from build123d import *

# Parameters (mm, degrees)
SKETCH3_R          = 1.75
CUT_EXTRUDE1_DEPTH = 10
SKETCH5_W          = 10
SKETCH5_H          = 10
CUT_EXTRUDE3_DEPTH = 50
CHAMFER1_START     = -23
CHAMFER1_2_DEPTH   = 2


with BuildPart() as part:
    # Sketch2 → Revolve1 (revolve)
    with BuildSketch(Plane.XY, mode=Mode.PRIVATE) as revolve1_sk:
        Polygon((25.1, 13), (27.1, 13), (27.1, -24), (37.1, -24), (37.1, -27), (24.1, -27), (24.1, -13), (25.1, -13), align=None)
    revolve(revolve1_sk.sketch.rotate(Axis((0, 0, 0), (0, -1, 0)), 90), axis=Axis((0, 0, 0), (0, -1, 0)))

    # Sketch3 → Cut-Extrude1 (cut)
    with BuildSketch(Plane(origin=(0, -24, 0), x_dir=(1, 0, 0), z_dir=(0, 1, 0))):
        with Locations(Location((-23.228457762, 23.228457762, 0), (0, 0, 270))):
            Circle(SKETCH3_R)
        with Locations(Location((23.228457762, 23.228457762, 0), (0, 0, 270))):
            Circle(SKETCH3_R)
        with Locations(Location((23.228457762, -23.228457762, 0), (0, 0, 270))):
            Circle(SKETCH3_R)
        with Locations(Location((-23.228457762, -23.228457762, 0), (0, 0, 270))):
            Circle(SKETCH3_R)
    extrude(amount=-CUT_EXTRUDE1_DEPTH, mode=Mode.SUBTRACT)

    # Sketch5 → Cut-Extrude3 (cut)
    with BuildSketch(Plane.XY):
        with Locations((0, -18)):
            Rectangle(SKETCH5_W, SKETCH5_H)
    extrude(amount=-CUT_EXTRUDE3_DEPTH, mode=Mode.SUBTRACT)

    # Chamfer1: read off the stored shape, not the designer's step
    # Chamfer1 outline → Chamfer1 (revolve)
    with BuildSketch(Plane.XY):
        Polygon((29.1, -24), (27.1, -22), (27.1, -24), align=None)
    revolve(axis=Axis((0, 0, 0), (0, 1, 0)))

    # Chamfer1 2 outline → Chamfer1 2 (cut)
    with BuildSketch(Plane(origin=(0, 0, 0), x_dir=(1, 0, 0), z_dir=(0, 1, 0)).offset(CHAMFER1_START)):
        with BuildLine():
            ThreePointArc((5, 27.651582233), (0, 28.1), (-5, 27.651582233))
            Line((-5, 27.651582233), (-5, 23.575623003))
            ThreePointArc((-5, 23.575623003), (0, 24.1), (5, 23.575623003))
            Line((5, 23.575623003), (5, 27.651582233))
        make_face()
    extrude(amount=CHAMFER1_2_DEPTH, mode=Mode.SUBTRACT)


solid = part.part
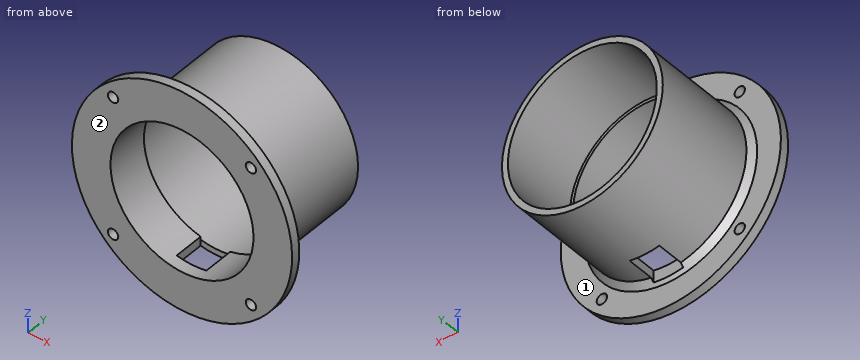
Design review of the part built by this model. Coordinates are the model's own, in mm. Face numbers are marked on the shaded views. A direction names the side the tool comes from. Coordinates: 2 decimals unless noted, no trailing zeros. Write each loop counter-clockwise with the first axis right and the second up, starting at its lowest first coordinate (ties: lowest second). Pieces come first, ordered by that corner, then holes. Notation, with made-up numbers: (83, -1.5) - (116, -1.5) arc R3 cw to (116, 2.5) - close; hole circle Ø2 at (-11, -21.5). An arc over 180 degrees is marked (long way). Use one line per item in the form item = value.
Q1. Consider section C-C (y = 1.5). Write out the cut boundary in (x, z).
Taken from the geometry:
outline = circle Ø54.2 at (0, 0); hole circle Ø50.2 at (0, 0)
Q2. Machinability: for the marked faces 1 and 2, which of the approach directions +Z, -Z, +X, -X, +Y, -Y give a long, thin tool a straight path to every point of the face, cutting with its end or side? Answer none if there is none.
Taken from the geometry:
face_1 = +Y
face_2 = +Z, -Z, +X, -X, -Y
Q3. Consider section B-B (x = 0). Write out the cut boundary in (y, z).
Taken from the geometry:
outline = (-27, -37.1) - (-24, -37.1) - (-24, -29.1) - (-23, -28.1) - (-23, -24.1) - (-27, -24.1) - close; (-27, 24.1) - (-13, 24.1) - (-13, 25.1) - (13, 25.1) - (13, 27.1) - (-22, 27.1) - (-24, 29.1) - (-24, 37.1) - (-27, 37.1) - close; (-13, -27.1) - (13, -27.1) - (13, -25.1) - (-13, -25.1) - close
Q4. Consider section A-A (z = 0). Write out the cut boundary in (x, y), plus the area to 3 significant figures.
Taken from the geometry:
outline = (-37.1, -27) - (-24.1, -27) - (-24.1, -13) - (-25.1, -13) - (-25.1, 13) - (-27.1, 13) - (-27.1, -22) - (-29.1, -24) - (-37.1, -24) - close; (24.1, -27) - (37.1, -27) - (37.1, -24) - (29.1, -24) - (27.1, -22) - (27.1, 13) - (25.1, 13) - (25.1, -13) - (24.1, -13) - close
area = 252 mm^2
Q5. For probe 1 along Z at (x, y) = (-0.5, -0.5); probe 2 along Y at (x, z) = (25, -23); probe 3 along X at (y, z) = (-20, -12.5), list the stretches that pass through material, from the lowest coordinate up.
Taken from the geometry:
probe_1 = -27.1 to -25.1, 25.1 to 27.1
probe_2 = -27 to -24
probe_3 = -24.04 to -20.6, 20.6 to 24.04
Q6. Insertion check: pin 1 Ø1.5 at (x, y) = (22.5, -4) entering from -Z; pin 2 Ø3 at (x, y) = (-19.5, -19) entering from +Z; pin 3 Ø4 at (x, z) = (-23.23, -23.23) entering from +Y. Each pin has a flat end and moves straight along its axis. Give the tip position at first contact, or say it passes through.
Taken from the geometry:
pin_1 = -16.17
pin_2 = 20.26
pin_3 = -24
Q7. Consider section D-D (y = -19). Write out the cut boundary in (x, z), plus the area to 3 significant figures.
Taken from the geometry:
outline = (-5, -26.63) - (-5, -23.58) arc R24.1 cw (long way) to (5, -23.58) - (5, -26.63) arc R27.1 ccw (long way) to start
area = 452 mm^2
